The listing builds one solid part. Answer for the finished solid, in the listing's coordinates (mm). Round coordinates to 2 decimals unless told otherwise and drop trailing zeros. Loops run counter-clockwise (first coordinate to the right, second up) from the corner with the lowest first, then second, coordinate; pieces in that order, holes last. Notation, with made-up numbers: (-38.75, 66) - (-2.75, 66) arc R20 ccw to (-2.75, 72) - close; hole circle Ø10 at (-9.5, 50.5). An arc over 180 degrees is marked (long way). One line per item, written item: value.
```python
from build123d import *

# Parameters (mm, degrees)
SKETCH5_W           = 45.93
SKETCH5_H           = 80
BOSS_EXTRUDE5_DEPTH = 3.1
SKETCH6_W           = 3.1
SKETCH6_H           = 39.153821237
BOSS_EXTRUDE6_DEPTH = 3.1
SKETCH7_R           = 9.525
CUT_EXTRUDE2_DEPTH  = 4.1


with BuildPart() as part:
    # Sketch5 → Boss-Extrude5 (new body)
    with BuildSketch(Plane.XY):
        Rectangle(SKETCH5_W, SKETCH5_H)
    extrude(amount=BOSS_EXTRUDE5_DEPTH)

    # Sketch6 → Boss-Extrude6 (add, through all)
    with BuildSketch(Plane.XY):
        with Locations((24.515, -20.423089381)):
            Rectangle(SKETCH6_W, SKETCH6_H)
        with Locations((-24.515, -20.423089381)):
            Rectangle(SKETCH6_W, SKETCH6_H)
    extrude(amount=BOSS_EXTRUDE6_DEPTH)

    # Sketch7 → Cut-Extrude2 (cut, through all)
    with BuildSketch(Plane.XY):
        Circle(SKETCH7_R)
        with BuildLine():
            Line((-15.470384182, 13.470384182), (-15.470384182, -13.470384182))
            Line((-15.470384182, -13.470384182), (-15.470384182, -18.470384182))
            ThreePointArc((-15.470384182, -18.470384182), (-13.470384182, -20.470384182), (-11.470384182, -18.470384182))
            Line((-11.470384182, -18.470384182), (-11.470384182, -13.470384182))
            Line((-11.470384182, -13.470384182), (-11.470384182, 13.470384182))
            Line((-11.470384182, 13.470384182), (-11.470384182, 18.470384182))
            ThreePointArc((-11.470384182, 18.470384182), (-13.470384182, 20.470384182), (-15.470384182, 18.470384182))
            Line((-15.470384182, 18.470384182), (-15.470384182, 13.470384182))
        make_face()
        with BuildLine():
            Line((11.470384182, 13.470384182), (11.470384182, 18.470384182))
            ThreePointArc((11.470384182, 18.470384182), (13.470384182, 20.470384182), (15.470384182, 18.470384182))
            Line((15.470384182, 18.470384182), (15.470384182, 13.470384182))
            Line((15.470384182, 13.470384182), (15.470384182, -13.470384182))
            Line((15.470384182, -13.470384182), (15.470384182, -18.470384182))
            ThreePointArc((15.470384182, -18.470384182), (13.470384182, -20.470384182), (11.470384182, -18.470384182))
            Line((11.470384182, -18.470384182), (11.470384182, -13.470384182))
            Line((11.470384182, -13.470384182), (11.470384182, 13.470384182))
        make_face()
    extrude(amount=CUT_EXTRUDE2_DEPTH, mode=Mode.SUBTRACT)


solid = part.part
```
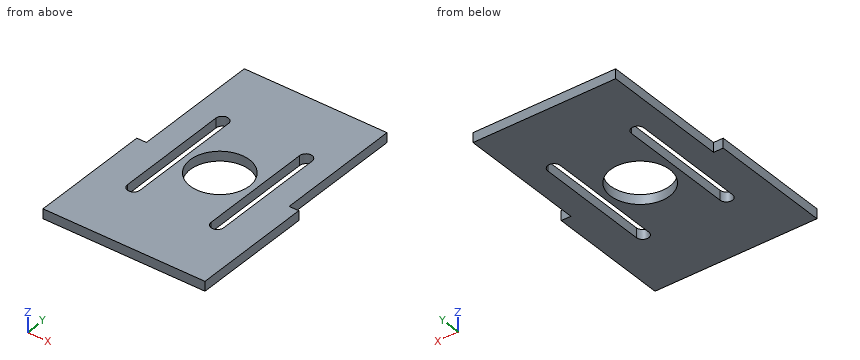
1) A cutting plane is placed at B-B on y = 0. Give the vertices of the cut face in (x, z) (3 decimals), and give its area (3 significant figures).
Final values:
outline: (-22.965, 0) - (-15.47, 0) - (-15.47, 3.1) - (-22.965, 3.1) - close; (-11.47, 0) - (-9.525, 0) - (-9.525, 3.1) - (-11.47, 3.1) - close; (9.525, 0) - (11.47, 0) - (11.47, 3.1) - (9.525, 3.1) - close; (15.47, 0) - (22.965, 0) - (22.965, 3.1) - (15.47, 3.1) - close
area: 58.5 mm2
2) Each of these flat-tipped pins is pushed along its axis until it touches: pin 1 Ø1.6 at (y, z) = (6, 1) entering from -X (3 decimals); pin 2 Ø1.6 at (x, z) = (-24.5, 1.5) entering from +Y. Where does it stop, or does it pass through?
Final values:
pin 1: x = -22.965
pin 2: y = -0.85
3) Consider L1, parallel to X at y = -16.5, z = 1.7 (3 decimals); L2, parallel to X at y = 0, z = 1.85 (3 decimals); L3, parallel to X at y = -2, z = 0.25 (3 decimals). Determine where each line is inside the solid, lowest interval first.
Final values:
L1: -26.065 to -15.47, -11.47 to 11.47, 15.47 to 26.065
L2: -22.965 to -15.47, -11.47 to -9.525, 9.525 to 11.47, 15.47 to 22.965
L3: -26.065 to -15.47, -11.47 to -9.313, 9.313 to 11.47, 15.47 to 26.065
4) A cutting plane is placed at A-A on z = 1.35. Give the vertices of the cut face in (x, y) (3 decimals), and give its area (3 significant figures).
Final values:
outline: (-26.065, -40) - (26.065, -40) - (26.065, -0.846) - (22.965, -0.846) - (22.965, 40) - (-22.965, 40) - (-22.965, -0.846) - (-26.065, -0.846) - close; hole (-15.47, -18.47) arc R2 ccw to (-11.47, -18.47) - (-11.47, 18.47) arc R2 ccw to (-15.47, 18.47) - close; hole circle Ø19.05 at (0, 0); hole (11.47, -18.47) arc R2 ccw to (15.47, -18.47) - (15.47, 18.47) arc R2 ccw to (11.47, 18.47) - close
area: 3,310 mm2
5) A cutting plane is placed at D-D on y = 11. Give the vertices of the cut face in (x, z) (3 decimals).
Final values:
outline: (-22.965, 0) - (-15.47, 0) - (-15.47, 3.1) - (-22.965, 3.1) - close; (-11.47, 0) - (11.47, 0) - (11.47, 3.1) - (-11.47, 3.1) - close; (15.47, 0) - (22.965, 0) - (22.965, 3.1) - (15.47, 3.1) - close
6) A cutting plane is placed at C-C on x = 12.5. Give the vertices of the cut face in (y, z), and give its area (3 significant figures).
Final values:
outline: (-40, 0) - (-20.22, 0) - (-20.22, 3.1) - (-40, 3.1) - close; (20.22, 0) - (40, 0) - (40, 3.1) - (20.22, 3.1) - close
area: 123 mm2
